Can you work these out from the drawing? Everything is in mm from the part's minimum corner. A direction names the side the tool comes from. Give positions to 0.01 mm unless a question says otherwise; leave off trailing zeros. Order: outer loops, then holes, each group sorted by start corner. A loop starts at its lowest first (then second) coordinate and runs counter-clockwise, first axis right, second up. Notation, with made-up numbers: M -33,-28.75 L 13,-28.75 A24 ccw 13,0.25 Z; hole C 13.5,-11.5 d3. An arc over 180 degrees is marked long. Answer in a Markdown table with one row per item. Add a question column.
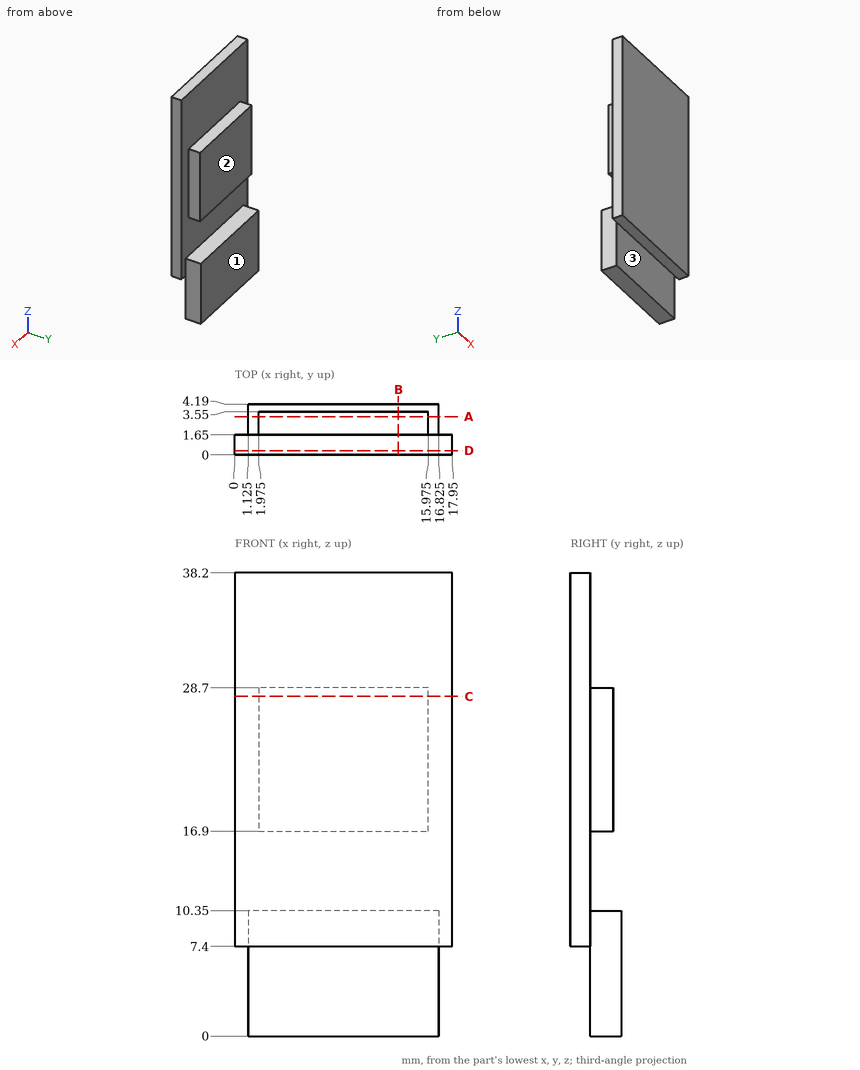
1. Suppose I cut it at A-A on y = 3.15. List the corners of the cut face in (x, z) for me (3 decimals).
2. Suppose I cut it at C-C on z = 28. List the corners of the cut face in (x, y) for me (3 decimals), plus the area to 3 significant figures.
3. Suppose I cut it at B-B on x = 13.5. List the corners of the cut face in (y, z) for me, plus the area to 3 significant figures.
4. For the marked faces 1, 2 and 3, which set-ups out of +Z, -Z, +X, -X, +Y, -Y let a thin tool reach every point of the face, with its end or its side?
5. If I drill on line 1 along Z through (x, y) = (6.5, 2.05); line 2 along X through (y, z) = (1.7, 26) (3 decimals); line 3 along Y through (x, z) = (11, 16.5), over which ranges is the centre line in solid material (lowest first)? Write a range as [from, to].
6. Will these pins go through, and if not, where does the flat tip stop? P1, Ø9.5, axis at x = 12, z = 25, coming from the +Y side; P2, Ø2, axis at y = 3.5, z = 7, coming from the +X side (3 decimals); P3, Ø4, axis at x = 2, z = 32, coming from the -Y side; P4, Ø8, axis at x = 11, z = 2, coming from the -Y side.
7. Suppose I cut it at D-D on y = 0.35. List the corners of the cut face in (x, z) for me.
Findings below:
| question | item | result |
|---|---|---|
| 1 | outline | M 1.125,0 L 16.825,0 L 16.825,10.35 L 1.125,10.35 Z; M 1.975,16.9 L 15.975,16.9 L 15.975,28.7 L 1.975,28.7 Z |
| 2 | outline | M 0,0 L 17.95,0 L 17.95,1.65 L 15.975,1.65 L 15.975,3.55 L 1.975,3.55 L 1.975,1.65 L 0,1.65 Z |
| 2 | area | 56.2 mm2 |
| 3 | outline | M 0,7.4 L 1.65,7.4 L 1.65,0 L 4.19,0 L 4.19,10.35 L 1.65,10.35 L 1.65,16.9 L 3.55,16.9 L 3.55,28.7 L 1.65,28.7 L 1.65,38.2 L 0,38.2 Z |
| 3 | area | 99.5 mm2 |
| 4 | face 1 | +Z, -Z, +X, -X, +Y |
| 4 | face 2 | +Z, +X, -X, +Y |
| 4 | face 3 | -Z, +X, -X, -Y |
| 5 | line 1 | [0, 10.35], [16.9, 28.7] |
| 5 | line 2 | [1.975, 15.975] |
| 5 | line 3 | [0, 1.65] |
| 6 | P1 | y = 3.55 |
| 6 | P2 | x = 16.825 |
| 6 | P3 | y = 0 |
| 6 | P4 | y = 1.65 |
| 7 | outline | M 0,7.4 L 17.95,7.4 L 17.95,38.2 L 0,38.2 Z |
